from build123d import *

# Parameters (mm, degrees)
F2_SIZE  = 0.5
F3_SIZE  = 0.5
F6_DEPTH = 3.9


with BuildPart() as f1:
    # F0 (on Front) → F1 (revolve)
    with BuildSketch(Plane.XZ):
        with BuildLine():
            add(Edge.make_bspline(
                [(1.5, 2.389568), (3.847685, 2.088384), (6.806025, 1.195458), (7.95, 0)],
                knots=[1.564524, 1.564524, 1.564524, 1.564524, 8.333817, 8.333817, 8.333817, 8.333817], degree=3))
            Line((7.95, 0), (10.65, 0))
            Line((10.65, 0), (10.65, 2.6))
            Line((10.65, 2.6), (6.05, 2.6))
            Line((6.05, 2.6), (6.05, 3))
            Line((6.05, 3), (4.05, 3))
            Line((4.05, 3), (4.05, 6.9))
            Line((4.05, 6.9), (0, 6.9))
            Line((0, 6.9), (0, 2.889568))
            Line((0, 2.889568), (1.5, 2.889568))
            Line((1.5, 2.889568), (1.5, 2.389568))
        make_face()
        with BuildLine():
            Line((0, 2.889568), (0, 2.5))
            add(Edge.make_bspline(
                [(0, 2.5), (0.447422, 2.497178), (0.957401, 2.459178), (1.5, 2.389568)],
                knots=[0, 0, 0, 0, 1.564524, 1.564524, 1.564524, 1.564524], degree=3))
            Line((1.5, 2.389568), (1.5, 2.889568))
            Line((1.5, 2.889568), (0, 2.889568))
        make_face()
    revolve(axis=Axis((0, 0, 3.45), (0, 0, -1)))

    # F2
    f2_edges = [f1.edges().sort_by_distance(p)[0] for p in [
        (-4.05, 0, 6.9),
    ]]
    chamfer(f2_edges, length=F2_SIZE)

    # F3
    f3_edges = [f1.edges().sort_by_distance(p)[0] for p in [
        (-10.65, 0, 0),
    ]]
    chamfer(f3_edges, length=F3_SIZE)

    # F5 (on offset) → F6 (cut)
    with BuildSketch(Plane.XY.offset(6.9)):
        with BuildLine():
            ThreePointArc((0.3, -2.984962), (2.22486, -2.012461), (3, 0))
            ThreePointArc((3, 0), (2.22486, 2.012461), (0.3, 2.984962))
            Line((0.3, 2.984962), (0.3, 0))
            Line((0.3, 0), (0.3, -2.984962))
        make_face()
        with BuildLine():
            Line((0.3, 0), (0.3, 2.984962))
            ThreePointArc((0.3, 2.984962), (0, 3), (-0.3, 2.984962))
            Line((-0.3, 2.984962), (-0.3, 0))
            Line((-0.3, 0), (0, 0))
            Line((0, 0), (0.3, 0))
        make_face()
        with BuildLine():
            ThreePointArc((-0.3, -2.984962), (0, -3), (0.3, -2.984962))
            Line((0.3, -2.984962), (0.3, 0))
            Line((0.3, 0), (0, 0))
            Line((0, 0), (-0.3, 0))
            Line((-0.3, 0), (-0.3, -2.984962))
        make_face()
        with BuildLine():
            Line((-0.3, 0), (-0.3, 2.984962))
            ThreePointArc((-0.3, 2.984962), (-3, 0), (-0.3, -2.984962))
            Line((-0.3, -2.984962), (-0.3, 0))
        make_face()
    extrude(amount=-F6_DEPTH, mode=Mode.SUBTRACT)


solid = f1.part
Verification items for the finished model (mm, model axes). A direction names the side the tool comes from. Give positions to 0.01 mm unless a question says otherwise; leave off trailing zeros. Order: outer loops, then holes, each group sorted by start corner. A loop starts at its lowest first (then second) coordinate and runs counter-clockwise, first axis right, second up. Notation, with made-up numbers: (22, 64.5) -> (73, 64.5) arc R22 ccw to (73, 88.5) -> close; hole circle Ø6 at (7.5, 0.25). An arc over 180 degrees is marked (long way). Answer as CSV lines item,"result".
Q1. Sectioned sample at A-A on z = 6. Record the cut outline in (x, y).
Solutions:
outline,"circle Ø8.1 at (0, 0); hole (-0.3, -2.98) arc R3 ccw to (0.3, -2.98) arc R3 ccw to (3, 0) arc R3 ccw to (0.3, 2.98) arc R3 ccw to (-0.3, 2.98) arc R3 ccw to start"
Q2. Release check for a two-part mould opening along Y. For faces 1 (the cylindrical face through (10.158, -3.199, 1.565)), 2 (the cylindrical face through (-3, 0, 5)), 3 (the flat face through (5, 5, 2.6)), 4 (the flat face through (0, 0, 3)) record: +Y half, -Y half, draft (parallel to the pull), parting line (faces both ways), or undercut.
Solutions:
face 1,"parting line"
face 2,"undercut"
face 3,"draft"
face 4,"undercut"
Q3. Scan lines: probe 1 along Z at (x, y) = (-1.25, 9.5); probe 2 along X at (y, z) = (0.75, 4.5); probe 3 along Y at (x, z) = (2.25, 4.25). Record each from-to range of solid material in increasing order.
Solutions:
probe 1,"z = 0 to 2.6"
probe 2,"x = -3.98 to -2.9, 2.9 to 3.98"
probe 3,"y = -3.37 to -1.98, 1.98 to 3.37"
Q4. Depth check by flat-ended pin: pin 1 (2 mm diameter, centred on y = 8, z = 3, fed in from -X); pin 2 (1.5 mm diameter, centred on y = 3.5, z = 4, fed in from +X); pin 3 (4 mm diameter, centred on y = -5.5, z = 1.5, fed in from -X). Enter the tip coordinate at first touch or a pass-through.
Solutions:
pin 1,"stops at x = -7.95"
pin 2,"stops at x = 2.97"
pin 3,"stops at x = -10.06"
Q5. Access from +Z, -Z, +X, -X, +Y, -Y to the whole of each face (thin tool, end or side, straight path). Record for faces 5 (the flat face through (6.8, 4.5, 0)), 6 (the flat face through (-1.43, 3.95, 3)).
Solutions:
face 5,"-Z, +X, -X, +Y, -Y"
face 6,"+Z"
